Geometry check sheet. Reference: the model listing, model coordinates, mm. A direction names the side the tool comes from. Round coordinates to 2 decimals unless told otherwise and drop trailing zeros. Order: outer loops, then holes, each group sorted by start corner. A loop starts at its lowest first (then second) coordinate and runs counter-clockwise, first axis right, second up.
(1) Sectioned sample at A-A (y = 10). Record the boundary of the cut face in (x, z).
(2) Set-up check for faces 5 (the face through (3.88, 32.11, -2.28)), 6 (the face through (-4, 20, 4)), 7 (the face through (-1.617, 4.481, -0.67)): record each of +Z, -Z, +X, -X, +Y, -Y from which the full face is reachable in a straight line by a thin tool's end or side.
(3) Go/stop test with flat-tipped pins: pin 1 (0.5 mm diameter, centred on x = 0.5, z = 5, fed in from +Y); pin 2 (1.5 mm diameter, centred on x = -6, z = -3.5, fed in from -Y); pin 3 (4 mm diameter, centred on y = 27, z = -5, fed in from -X). Record where each tip stops, or that it passes through.
(4) Material ranges on line 1 along X through (y, z) = (4, 0); line 2 along Z through (x, y) = (-1.5, 10); line 3 along X through (y, z) = (8, -1.25), recorded low to high.
(5) Release check for a two-part mould opening along X. For faces 1 (the face through (-0.066, 14.869, -0.297)), 2 (the face through (3.98, 39.86, 2.38)), 3 (the face through (-4.05, 39.86, 2.26)), 4 (the face through (2, 0, 0)) record: +X half, -X half, draft (parallel to the pull), parting line (faces both ways), or undercut.
from build123d import *

# Parameters (mm, degrees)
F0_R            = 8
F1_DEPTH        = 20
F2_R            = 5
F3_DEPTH        = 20
F5_DEPTH        = 16
F5_COPIES_COUNT = 3
F6_SIZE         = 0.49999
F7_R            = 0.5
F9_D            = 3.5
F9_DEPTH        = 14
F9_TIP          = 1.0515060833
F10_R           = 2.1
F11_DEPTH       = 8.25
F12_SIZE        = 3


# Not quite as in the source:
# - a fillet or chamfer is up to 0.001 mm smaller than in the source, because OpenCascade refuses the exact size
# - a pattern or mirror of a feature is missing from the dataset's text; its kind, count and spacing are read off the source's solid


with BuildPart() as f1:
    # F0 (on Front) → F1 (new body)
    with BuildSketch(Plane.XZ):
        Circle(F0_R)
    extrude(amount=-F1_DEPTH)

    # F2 (on face) → F3 (join)
    with BuildSketch(Plane(origin=(0, 20, 0), x_dir=(-1, 0, 0), z_dir=(0, 1, 0))):
        Circle(F2_R)
    extrude(amount=F3_DEPTH)

    # F4 (on face) → F5 (cut)
    with BuildSketch(Plane(origin=(0, 40, 0), x_dir=(-1, 0, 0), z_dir=(0, 1, 0))):
        with BuildLine():
            ThreePointArc((2.1794494718, 4.5), (0, 5), (-2.1794494718, 4.5))
            Line((-2.1794494718, 4.5), (2.1794494718, 4.5))
        make_face()
    f5 = extrude(amount=-F5_DEPTH, mode=Mode.SUBTRACT)

    # F5_copies: F5 ×3 about axis
    f5_copies_axis = Axis((0, 0, 0), (0, 1, 0))
    for i in range(1, F5_COPIES_COUNT):
        add(f5.rotate(f5_copies_axis, i * 360 / F5_COPIES_COUNT), mode=Mode.SUBTRACT)

    # F6 (size 0.5 in the source; OpenCascade refuses exactly that, so slightly less here)
    f6_edges = [f1.edges().sort_by_distance(p)[0] for p in [
        (4.330127, 40, 2.5),
        (-4.996709, 40, -0.18139),
        (0, 40, -5),
        (-4.236582, 40, 2.655443),
    ]]
    chamfer(f6_edges, length=F6_SIZE)

    # F7
    f7_edges = [f1.edges().sort_by_distance(p)[0] for p in [
        (-8, 20, 0),
        (5, 20, 0),
    ]]
    fillet(f7_edges, radius=F7_R)

    # F9
    with Locations(Plane.XZ):
        with Locations((0, 0)):
            Hole(F9_D / 2, depth=F9_DEPTH)
            with Locations((0, 0, -(F9_DEPTH + F9_TIP / 2))):  # 118° drill point
                Cone(0, F9_D / 2, F9_TIP, mode=Mode.SUBTRACT)

    # F10 (on Right) → F11 (cut, symmetric)
    with BuildSketch(Plane.YZ):
        with Locations((10, 0)):
            Circle(F10_R)
    extrude(amount=F11_DEPTH, both=True, mode=Mode.SUBTRACT)

    # F12
    f12_edges = [f1.edges().sort_by_distance(p)[0] for p in [
        (-8, 0, 0),
    ]]
    chamfer(f12_edges, length=F12_SIZE)


solid = f1.part
Answer below:
1. outline: (-7.72, -2.1) arc R8 ccw to (7.72, -2.1) - close; (-7.72, 2.1) - (7.72, 2.1) arc R8 ccw to start
2. face 5: -Z, +X, +Y
2. face 6: +Y
2. face 7: -Y
3. pin 1: stops at y = 24
3. pin 2: stops at y = 1.2
3. pin 3: stops at x = -3.46
4. line 1: x = -8 to -1.75, 1.75 to 8
4. line 2: z = -7.86 to -2.1, 2.1 to 7.86
4. line 3: x = -7.9 to -1.22, 1.22 to 7.9
5. face 1: undercut
5. face 2: +X half
5. face 3: -X half
5. face 4: draft
